The listing builds one solid part. Answer for the finished solid, in the listing's coordinates (mm). A direction names the side the tool comes from. Round coordinates to 2 decimals unless told otherwise and drop trailing zeros. Loops run counter-clockwise (first coordinate to the right, second up) from the corner with the lowest first, then second, coordinate; pieces in that order, holes last. Notation, with made-up numbers: (69, 19) -> (104, 19) arc R33 ccw to (104, 48) -> close; hole circle Ø3 at (43, 2). An arc over 180 degrees is marked (long way). Write each question's results on one line, items separated by ' | '. Start each with the question number.
(1) The part is cut by section A-A (z = -19). Determine the outline of the cut face in (x, y) (3 decimals), plus the area to 3 significant figures.
(2) Determine the mould class of faces 4 (the face through (-6.5, 12, -16)), 5 (the face through (3.2, 13.5, 3.2)), 6 (the face through (-1.379, 6.833, 3.325)) for opening direction X: released by +X, released by -X, zero draft, split by the parting line, or undercut.
(3) Straight lines are drawn through the part: probe 1 along Y at (x, z) = (-7.1, -19); probe 2 along X at (y, z) = (13.2, 0); probe 3 along Y at (x, z) = (-2, -19) (3 decimals). For each, find the intervals that lie inside material, in ascending order.
(4) The part is cut by section C-C (y = 15.25). Determine the outline of the cut face in (x, z).
(5) The part is cut by section B-B (x = 1.5). Count the separate pieces of the cut face and the enclosed holes in it, plus the area to 3 significant figures.
(6) For faces 1 (the face through (-6.9, 12.3, -20.5)), 2 (the face through (6.88, 12.18, -20.75)), 3 (the face through (0, 14, -9)), determine the directions among +Z, -Z, +X, -X, +Y, -Y from which every point of the face is accessible in a straight line to the end or side of a thin tool.
(7) Flat-ended cylindrical pins translate along their axes: pin 1 (4.5 mm diameter, centred on x = 2.5, z = 1.5, fed in from +Y); pin 2 (4.5 mm diameter, centred on x = 0, z = 0, fed in from -Y); pin 3 (1 mm diameter, centred on x = -3, y = 0.5, fed in from +Z); pin 4 (3.5 mm diameter, centred on x = -1.5, y = -1.5, fed in from +Z). Find the tip coordinate at first contact, or state that the pin passes through.
```python
from build123d import *

# Parameters (mm, degrees)
EXTRUDE_1_DEPTH      = 11
EXTRUDE_2_DEPTH      = 3
EXTRUDE_2_DEPTH_BACK = 16.5
FILLET_1_R           = 1
SKETCH_6_W           = 1
SKETCH_6_H           = 1
CUT_EXTRUDE_3_DEPTH  = 10
CUT_EXTRUDE_4_REACH  = 63.673
SKETCH_8_R           = 0.5
SKETCH_9_R           = 1.5
CUT_EXTRUDE_5_DEPTH  = 1
SKETCH_10_R          = 1.75
CUT_EXTRUDE_6_DEPTH  = 1
FILLET_2_R           = 0.25
SKETCH_11_R          = 2
CUT_EXTRUDE_7_DEPTH  = 13.5
SKETCH_13_R          = 3.6
CUT_EXTRUDE_8_DEPTH  = 13.5
SKETCH_14_R          = 4.3
CUT_EXTRUDE_9_DEPTH  = 0.8
CUT_EXTRUDE_START    = -0.8
SKETCH_15_R          = 4.3
CUT_EXTRUDE_10_DEPTH = 0.8
SKETCH_16_R          = 0.875
CUT_EXTRUDE_11_DEPTH = 13


with BuildPart() as part:
    # 스케치1 → 보스-돌출1 (new body)
    with BuildSketch(Plane(origin=(0, 0, 0), x_dir=(1, 0, 0), z_dir=(0, 1, 0))):
        with BuildLine():
            Line((-7.5, 0), (-7.5, 50))
            ThreePointArc((-7.5, 50), (0, 57.5), (7.5, 50))
            Line((7.5, 50), (7.5, 0))
            ThreePointArc((7.5, 0), (0, -7.5), (-7.5, 0))
        make_face()
    extrude(amount=EXTRUDE_1_DEPTH)

    # 스케치2 → 회전1 (revolve)
    with BuildSketch(Plane.XY):
        Polygon((-7.5, 11), (0, 11), (0, 13.5), (-7.5, 13.5), (-6.5, 12.25), align=None)
    revolve(axis=Axis((0, 13.5, 0), (0, -1, 0)))

    # 스케치3 → 보스-돌출2 (add, two sides: drawn at the far end of the back side and taken through both)
    with BuildSketch(Plane.XZ.offset(-EXTRUDE_2_DEPTH_BACK)):
        with BuildLine():
            Line((-7.5, -50), (-7.5, -9))
            Line((-7.5, -9), (7.5, -9))
            Line((7.5, -9), (7.5, -50))
            ThreePointArc((7.5, -50), (0, -57.5), (-7.5, -50))
        make_face()
    extrude(amount=EXTRUDE_2_DEPTH + EXTRUDE_2_DEPTH_BACK)

    # 필렛1
    fillet_1_edges = [part.edges().sort_by_distance(p)[0] for p in [
        (7.5, -1.5, -9),
        (-7.5, -1.5, -9),
        (7.5, 13.75, -9),
        (-7.5, 13.75, -9),
    ]]
    fillet(fillet_1_edges, radius=FILLET_1_R)

    # 스케치6 → 컷-돌출3 (cut)
    with BuildSketch(Plane.XY.offset(-9)):
        with Locations((-7, 12.25)):
            Rectangle(SKETCH_6_W, SKETCH_6_H)
        with Locations((7, 12.25)):
            Rectangle(SKETCH_6_W, SKETCH_6_H)
    extrude(amount=-CUT_EXTRUDE_3_DEPTH, mode=Mode.SUBTRACT)

    # 컷-돌출4: up to this face of the body (flat: up to its plane)
    cut_extrude_4_end = Plane(part.part.faces().sort_by_distance((7.5, 6.537741203, -27.036889898))[0])
    # 스케치8 → 컷-돌출4 (cut, up to the picked face)
    with BuildSketch(Plane.ZY.offset(7.5), mode=Mode.PRIVATE) as cut_extrude_4_sk1:
        with Locations(Location((-19, 12.25, 0), (0, 0, 270))):
            Circle(SKETCH_8_R)
    cut_extrude_4_tool1 = split(extrude(cut_extrude_4_sk1.sketch, amount=-CUT_EXTRUDE_4_REACH, mode=Mode.PRIVATE), bisect_by=cut_extrude_4_end, keep=Keep.BOTH, mode=Mode.PRIVATE)
    add(cut_extrude_4_tool1.solids().sort_by(Axis((-7.5, 12.25, -19), (1, 0, 0)))[0], mode=Mode.SUBTRACT)

    # 스케치9 → 컷-돌출5 (cut)
    with BuildSketch(Plane.ZY.offset(7.5)):
        with Locations((-19, 12.25)):
            Circle(SKETCH_9_R)
    extrude(amount=-CUT_EXTRUDE_5_DEPTH, mode=Mode.SUBTRACT)

    # 스케치10 → 컷-돌출6 (cut)
    with BuildSketch(Plane(origin=(7.5, 0, 0), x_dir=(0, 0, -1), z_dir=(1, 0, 0))):
        with Locations((19, 12.25)):
            Circle(SKETCH_10_R)
    extrude(amount=-CUT_EXTRUDE_6_DEPTH, mode=Mode.SUBTRACT)

    # 필렛2
    fillet_2_edges = [part.edges().sort_by_distance(p)[0] for p in [
        (7.207106781, 12.75, -9.292893219),
        (7.207106781, 11.75, -9.292893219),
        (-7.5, 11.75, -13.792893219),
        (-7.5, 12.75, -13.792893219),
        (-7.5, 12.25, -20.5),
        (7.5, 12.75, -13.661474508),
        (7.5, 11.75, -13.661474508),
        (7.5, 12.25, -20.75),
        (-7.207106781, 11.75, -9.292893219),
        (-7.207106781, 12.75, -9.292893219),
    ]]
    fillet(fillet_2_edges, radius=FILLET_2_R)

    # 스케치11 → 컷-돌출7 (cut)
    with BuildSketch(Plane(origin=(0, 13.5, 0), x_dir=(1, 0, 0), z_dir=(0, 1, 0))):
        with Locations(Location((0, 0, 0), (0, 0, 270))):
            Circle(SKETCH_11_R)
    extrude(amount=-CUT_EXTRUDE_7_DEPTH, mode=Mode.SUBTRACT)

    # 스케치13 → 컷-돌출8 (cut)
    with BuildSketch(Plane(origin=(0, 13.5, 0), x_dir=(1, 0, 0), z_dir=(0, 1, 0))):
        with Locations(Location((0, 0, 0), (0, 0, 270))):
            Circle(SKETCH_13_R)
    extrude(amount=-CUT_EXTRUDE_8_DEPTH, mode=Mode.SUBTRACT)

    # 스케치14 → 컷-돌출9 (cut)
    with BuildSketch(Plane(origin=(0, 13.5, 0), x_dir=(1, 0, 0), z_dir=(0, 1, 0))):
        with Locations(Location((0, 0, 0), (0, 0, 270))):
            Circle(SKETCH_14_R)
    extrude(amount=-CUT_EXTRUDE_9_DEPTH, mode=Mode.SUBTRACT)

    # 스케치15 → 컷-돌출10 (cut)
    with BuildSketch(Plane(origin=(0, 0, 0), x_dir=(-1, 0, 0), z_dir=(0, -1, 0)).offset(CUT_EXTRUDE_START)):
        with Locations(Location((0, 0, 0), (0, 0, 270))):
            Circle(SKETCH_15_R)
    extrude(amount=CUT_EXTRUDE_10_DEPTH, mode=Mode.SUBTRACT)

    # 스케치16 → 컷-돌출11 (cut)
    with BuildSketch(Plane(origin=(6.5, 0, 0), x_dir=(0, 0, -1), z_dir=(1, 0, 0))):
        with Locations((19, 12.25)):
            Circle(SKETCH_16_R)
    extrude(amount=-CUT_EXTRUDE_11_DEPTH, mode=Mode.SUBTRACT)


solid = part.part
```
Checked values:
1) outline: (-7.5, -3) -> (7.5, -3) -> (7.5, 10.25) arc R0.25 ccw to (7.25, 10.5) -> (6.5, 10.5) -> (6.5, 11.375) -> (-6.5, 11.375) -> (-6.5, 10.75) -> (-7.25, 10.75) arc R0.25 ccw to (-7.5, 10.5) -> close; (-7.5, 14) arc R0.25 ccw to (-7.25, 13.75) -> (-6.5, 13.75) -> (-6.5, 13.125) -> (6.5, 13.125) -> (6.5, 14) -> (7.25, 14) arc R0.25 ccw to (7.5, 14.25) -> (7.5, 16.5) -> (-7.5, 16.5) -> close | area: 263 mm2
2) face 4: released by -X | face 5: zero draft | face 6: undercut
3) probe 1: y = -3 to 10.75, 13.75 to 16.5 | probe 2: x = -7.26 to -4.3, 4.3 to 7.26 | probe 3: y = -3 to 11.375, 13.125 to 16.5
4) outline: (-7.5, -50) arc R7.5 ccw to (7.5, -50) -> (7.5, -10) arc R1 ccw to (6.5, -9) -> (-6.5, -9) arc R1 ccw to (-7.5, -10) -> close
5) separate pieces: 2 | enclosed holes: 1 | area: 1,060 mm2
6) face 1: -X | face 2: +X | face 3: +X, -X, +Y
7) pin 1: stops at y = 13.5 | pin 2: passes through | pin 3: stops at z = 7.07 | pin 4: stops at z = 7.48
